```python
from build123d import *

# Parameters (mm, degrees)
F0_R          = 11.1125
F0_R_2        = 7.9375
F1_DEPTH      = 203.2
F1_DEPTH_BACK = 50.8
F2_R          = 7.9375
F3_DEPTH      = 6.35
F4_R          = 3.175


with BuildPart() as f1:
    # F0 (on Top) → F1 (new body, two sides)
    with BuildSketch(Plane.XY) as f1_sk:
        Circle(F0_R)
        Circle(F0_R_2, mode=Mode.SUBTRACT)
    extrude(amount=F1_DEPTH)
    extrude(f1_sk.sketch, amount=-F1_DEPTH_BACK)

    # F2 (on Top) → F3 (join)
    with BuildSketch(Plane.XY):
        with BuildLine():
            ThreePointArc((25.4, 23.8125), (24.935032, 24.935032), (23.8125, 25.4))
            Line((23.8125, 25.4), (-23.8125, 25.4))
            ThreePointArc((-23.8125, 25.4), (-24.935032, 24.935032), (-25.4, 23.8125))
            Line((-25.4, 23.8125), (-25.4, -23.8125))
            ThreePointArc((-25.4, -23.8125), (-24.935032, -24.935032), (-23.8125, -25.4))
            Line((-23.8125, -25.4), (23.8125, -25.4))
            ThreePointArc((23.8125, -25.4), (24.935032, -24.935032), (25.4, -23.8125))
            Line((25.4, -23.8125), (25.4, 23.8125))
        make_face()
        Circle(F2_R, mode=Mode.SUBTRACT)
    extrude(amount=F3_DEPTH)

    # F4
    f4_edges = [f1.edges().sort_by_distance(p)[0] for p in [
        (-11.1125, 0, 6.35),
    ]]
    fillet(f4_edges, radius=F4_R)


solid = f1.part
```
The model under review builds one solid part; all positions refer to its coordinate system, in mm. A direction names the side the tool comes from. Coordinates: 2 decimals unless noted, no trailing zeros. Write each loop counter-clockwise with the first axis right and the second up, starting at its lowest first coordinate (ties: lowest second). Pieces come first, ordered by that corner, then holes. Notation, with made-up numbers: (-28, 36) -> (19, 36) arc R21 cw to (19, 67) -> close; hole circle Ø6 at (-32, 39). An arc over 180 degrees is marked (long way). One line per item, written item: value. Start each with the question number.
Q1. Clearance check with flat-ended pins moving along their axes: P1, Ø5, axis at y = -1, z = 42.5, coming from the -X side; P2, Ø10, axis at x = -6.5, y = 17, coming from the +Z side; P3, Ø4, axis at x = -4, z = 72, coming from the -Y side; P4, Ø14.5, axis at x = 0, y = 0, coming from the -Z side. State where each tip first meets the part, or that it passes through.
Q2. For faces 4 (the face through (10.6, 3.34, -25.04)), 5 (the face through (11, -11, 6.35)), 6 (the face through (0, 25.4, 3)), list the 3-axis set-ups (+Z, -Z, +X, -X, +Y, -Y) from which the entire face can be reached by the end or side of a thin tool; tool diameter is ignored.
Q3. To check wall thickness, follow probe 1 along Y at (x, z) = (0, 131.5); probe 2 along Y at (x, z) = (0, 4.5); probe 3 along Z at (x, y) = (3.5, 20.5). State the ranges of each line that lie inside material, in increasing order.
Q4. The part is to be moulded in two halves that separate along Y. For faces 1 (the face through (-1.72, -7.75, 77.98)), 2 (the face through (-8, 3, 203.2)), 3 (the face through (10.6, 3.34, 107.72)), say which applies: +Y half, -Y half, draft (parallel to the pull), parting line (faces both ways), or undercut.
Q5. Add section D-D, the plane y = -18. Give the boundary of the cut face in (x, z), then the cut area to 3 significant figures.
Q6. Add section C-C, the plane z = 19. Give the boundary of the cut face in (x, y) (1 decimal), then the cut area to 3 significant figures.
Response:
1. P1: x = -11.11
1. P2: z = 6.54
1. P3: y = -10.93
1. P4: through
2. face 4: -Z
2. face 5: +Z
2. face 6: +Z, -Z, +X, -X, +Y
3. probe 1: -11.11 to -7.94, 7.94 to 11.11
3. probe 2: -25.4 to -7.94, 7.94 to 25.4
3. probe 3: 0 to 6.35
4. face 1: undercut
4. face 2: draft
4. face 3: parting line
5. outline: (-25.4, 0) -> (25.4, 0) -> (25.4, 6.35) -> (-25.4, 6.35) -> close
5. area: 323 mm²
6. outline: circle Ø22.2 at (0, 0); hole circle Ø15.9 at (0, 0)
6. area: 190 mm²
